Verification items for this drawing (mm, ordinates from the low corner). Give positions to 0.01 mm unless a question says otherwise; leave off trailing zeros. Order: outer loops, then holes, each group sorted by start corner. A loop starts at its lowest first (then second) coordinate and runs counter-clockwise, first axis right, second up. Notation, with made-up numbers: (79, -32.5) -> (99, -32.5) arc R22 cw to (99, -4.5) -> close; hole circle Ø5 at (21.25, -12.75). An arc over 180 degrees is marked (long way). One line per question, with ' | ' between items.
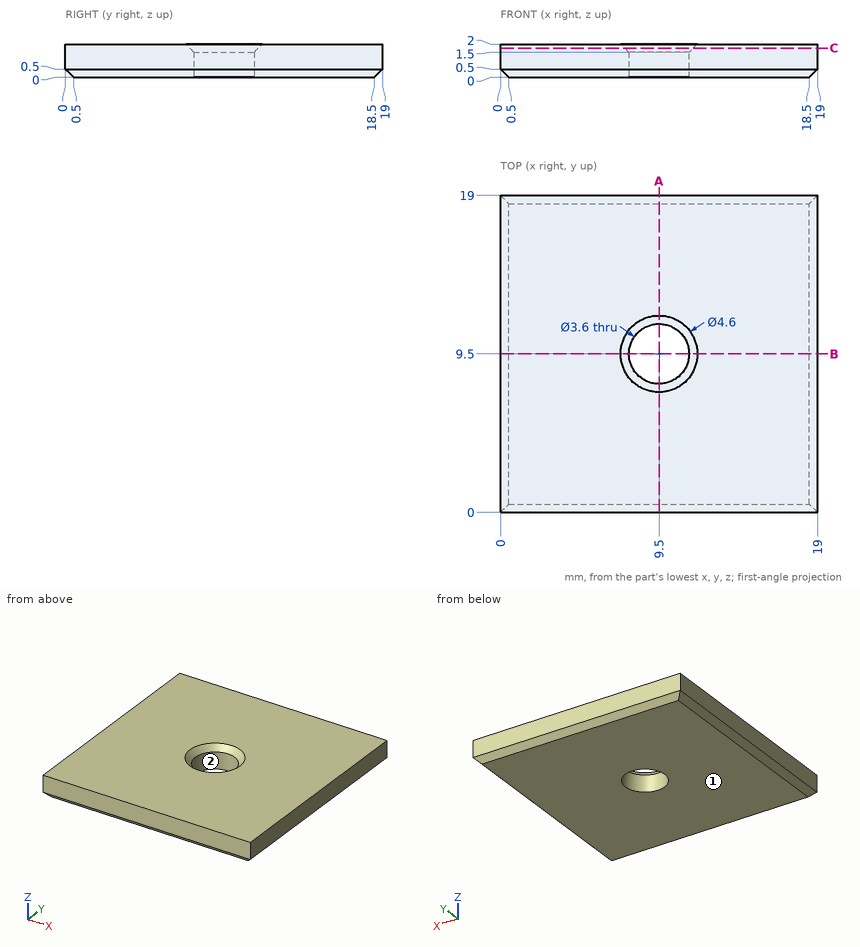
Q1. Section check C-C (z = 1.75). Enter the section's corners in (x, y).
Result sheet:
outline: (0, 0) -> (19, 0) -> (19, 19) -> (0, 19) -> close; hole circle Ø4.1 at (9.5, 9.5)
Q2. Mould release check, pull along X, two halves, no side actions. Record for the marked faces 1 and 2: pulls with the +X half, pulls with the -X half, needs draft (parallel to the pull), parting line crosses it, or undercut.
Result sheet:
face 1: needs draft | face 2: undercut
Q3. Thickness scan on line 1 (Y direction, x = 9.5, z = 1.25); line 2 (Y direction, x = 8, z = 1.05). Record the ranges inside material, lowest first.
Result sheet:
line 1: y = 0 to 7.7, 11.3 to 19 | line 2: y = 0 to 8.51, 10.49 to 19
Q4. Section check A-A (x = 9.5). Enter the section's corners in (y, z).
Result sheet:
outline: (0, 0.5) -> (0.5, 0) -> (7.7, 0) -> (7.7, 1.5) -> (7.2, 2) -> (0, 2) -> close; (11.3, 0) -> (18.5, 0) -> (19, 0.5) -> (19, 2) -> (11.8, 2) -> (11.3, 1.5) -> close
